```python
from build123d import *

# Parameters (mm, degrees)
F1_DEPTH = 10
F3_DEPTH = 4
F5_DEPTH = 50
F6_R     = 65
F7_DEPTH = 15
F8_DEPTH = 50
F9_DEPTH = 4


with BuildPart() as f1:
    # F0 (on Top) → F1 (new body)
    with BuildSketch(Plane.XY):
        with BuildLine():
            ThreePointArc((-78.2623792125, 110), (-135, 0), (-78.2623792125, -110))
            Line((-78.2623792125, -110), (78.2623792125, -110))
            ThreePointArc((78.2623792125, -110), (135, 0), (78.2623792125, 110))
            Line((78.2623792125, 110), (-78.2623792125, 110))
        make_face()
    extrude(amount=F1_DEPTH)

    # F2 (on face) → F3 (cut)
    with BuildSketch(Plane.XY.offset(10)):
        with BuildLine():
            Line((-61.4491659829, 110), (-69.2820323028, 110))
            ThreePointArc((-69.2820323028, 110), (-130, 0), (-69.2820323028, -110))
            Line((-69.2820323028, -110), (-61.4491659829, -110))
            ThreePointArc((-61.4491659829, -110), (-126, 0), (-61.4491659829, 110))
        make_face()
        with BuildLine():
            Line((69.2820323028, 110), (61.4491659829, 110))
            ThreePointArc((61.4491659829, 110), (126, 0), (61.4491659829, -110))
            Line((61.4491659829, -110), (69.2820323028, -110))
            ThreePointArc((69.2820323028, -110), (130, 0), (69.2820323028, 110))
        make_face()
    extrude(amount=-F3_DEPTH, mode=Mode.SUBTRACT)

    # F5 (add): faces of the model
    f5_faces = [f1.faces().sort_by_distance(p)[0] for p in [
        (-65.3655991429, 109.7695673269, 6),
        (128.3043267313, 0, 6),
    ]]
    extrude(f5_faces, amount=F5_DEPTH)

    # F6 (on face) → F7 (join)
    with BuildSketch(Plane(origin=(0, 0, 0), x_dir=(1, 0, 0), z_dir=(0, 0, -1))):
        with Locations((60.9998414516, 0)):
            Circle(F6_R)
    extrude(amount=F7_DEPTH)

    # F8 (cut): faces of the model
    f8_faces = [f1.faces().sort_by_distance(p)[0] for p in [
        (-65.3655991429, 109.7695673269, 56),
        (128.3043267313, 0, 56),
    ]]
    extrude(f8_faces, amount=-F8_DEPTH, mode=Mode.SUBTRACT)

    # F9 (add): faces of the model
    f9_faces = [f1.faces().sort_by_distance(p)[0] for p in [
        (-65.3655991429, 109.7695673269, 6),
        (128.3043267313, 0, 6),
    ]]
    extrude(f9_faces, amount=F9_DEPTH)


solid = f1.part
```
CAD build for the part. Positions are in the model's coordinates, mm. A direction names the side the tool comes from. Round coordinates to 2 decimals unless told otherwise and drop trailing zeros. Order: outer loops, then holes, each group sorted by start corner. A loop starts at its lowest first (then second) coordinate and runs counter-clockwise, first axis right, second up. Notation, with made-up numbers: (59, 15) -> (76, 15) arc R25 cw to (76, 33) -> close; hole circle Ø7 at (60, 2.25). An arc over 180 degrees is marked (long way). Write item = value, one per line.
(1) 3-axis set-ups, long thin cutter, end or side, ignore diameter. For faces 1 (the cylindrical face through (-134.988, 1.8, 4.93)), 2 (the cylindrical face through (123, -19.52, -7.4)): which of +Z, -Z, +X, -X, +Y, -Y reach the whole face in a straight line?
Answers follow:
face_1 = +Z, -Z, -X
face_2 = -Z
(2) Drill centre lines: L1, parallel to Z at x = 36, y = -101; L2, parallel to Y at x = 107.5, z = 1.25; L3, parallel to X at y = -23, z = 6.5. Where is each one in solid material? Low to high.
Answers follow:
L1 = 0 to 10
L2 = -81.66 to 81.66
L3 = -133.03 to 133.03
(3) Cut at D-D (y = -23.5). Write the cut outline in (x, z).
Answers follow:
outline = (-132.94, 0) -> (0.4, 0) -> (0.4, -15) -> (121.6, -15) -> (121.6, 0) -> (132.94, 0) -> (132.94, 10) -> (-132.94, 10) -> close
(4) Flat gauge pins, fed straight in: P1, Ø1, axis at x = 26.5, z = -12, coming from the -Y side; P2, Ø4, axis at x = 16.5, z = -11.5, coming from the +Y side; P3, Ø10, axis at x = -22.5, z = -9.5, coming from the -Y side; P4, Ø6, axis at x = 4, z = -9.5, coming from the +Y side. Where does each tip first touch, or does it go through?
Answers follow:
P1 = -55.4
P2 = 49.18
P3 = through
P4 = 36.18
(5) Cut at A-A (y = 0). Write the cut outline in (x, z).
Answers follow:
outline = (-135, 0) -> (-4, 0) -> (-4, -15) -> (126, -15) -> (126, 0) -> (135, 0) -> (135, 10) -> (-135, 10) -> close
(6) Cut at B-B (z = -6.5). Write the cut outline in (x, y).
Answers follow:
outline = circle Ø130 at (61, 0)
(7) Cut at C-C (x = -83.5). Write the cut outline in (y, z).
Answers follow:
outline = (-106.08, 0) -> (106.08, 0) -> (106.08, 10) -> (-106.08, 10) -> close
